Autodesk Inventor part; units mm, degrees
ref_plane "YZ Plane" through (0, 0, 0) normal (1, 0, 0) x (0, 1, 0)
ref_plane "XZ Plane" through (0, 0, 0) normal (0, 1, 0) x (-1, 0, 0)
ref_plane "XY Plane" through (0, 0, 0) normal (0, 0, 1) x (1, 0, 0)
sketch "Sketch1" plane through (0, 0, 0) normal (0, 1, 0) x (-1, 0, 0)
  circle A0 centre (-34.3765, 114.6665) radius 1.6
  circle A1 centre (-34.8464, 1.7591) radius 1.6
  arc A2 (-53.1019, 117.2341) -> (-38.3819, -1.7764) centre (30.561, 67.1665) ccw
  line L0 (-34.3765, 119.6665) -> (-48.8115, 119.6665)
  arc A3 (-38.3819, -1.7764) -> (-36.4764, -3.6306) centre (30.561, 67.1665) ccw
  line L1 (-33.0386, -5) -> (-21.9122, -5)
  line L2 (-16.9122, 0.0037) -> (-16.9963, 114.6702)
  line L3 (-21.9963, 119.6665) -> (-34.3765, 119.6665)
  arc A4 (-48.8115, 119.6665) -> (-53.1019, 117.2341) centre (-48.8115, 114.6665) ccw
  arc A5 (-36.4764, -3.6306) -> (-33.0386, -5) centre (-33.0386, 0) ccw
  circle A6 centre (-22.239, 104.2134) radius 1.25
  circle A7 centre (-53.239, 104.2134) radius 1.25
  circle A8 centre (-53.239, 29.2134) radius 1.25
  circle A9 centre (-22.239, 29.2134) radius 1.25
  line L4 (-24.639, 102.8634) -> (-24.639, 30.5634)
  line L5 (-24.639, 30.5634) -> (-51.939, 30.5634)
  line L6 (-51.939, 30.5634) -> (-51.939, 102.8634)
  line L7 (-51.939, 102.8634) -> (-24.639, 102.8634)
  arc A10 (-21.9122, -5) -> (-16.9122, 0.0037) centre (-21.9122, 0) ccw
  arc A11 (-16.9963, 114.6702) -> (-21.9963, 119.6665) centre (-21.9963, 114.6665) ccw
  point P0 (0, 0)
extrude "Extrusion1" add sketch "Sketch1" along normal blind 3
properties part number "LCD Plate" material "Polycarbonate, Clear"
Geometry: final body of the model. Coordinates: model frame, mm. A direction names the side the tool comes from. Round coordinates to 2 decimals unless told otherwise and drop trailing zeros. Loops run counter-clockwise (first coordinate to the right, second up) from the corner with the lowest first, then second, coordinate; pieces in that order, holes last.
Q1. Section A-A on z = 98.5. Return loops of the section in (x, y).
Q2. Pull-direction query (Z, two-part tool) for faces 3 (the cylindrical face through (34.864, 1.479, -4.655)), 4 (the cylindrical face through (66.086, 1.479, 54.302)), 5 (the cylindrical face through (53.51, 1.479, 105.434)); classes: released by +Z, released by -Z, zero draft, split by the parting line, or undercut.
Q3. Material intervals for L1, parallel to X at y = 1.9, z = 30; L2, parallel to X at y = 1.55, z = 103.5; L3, parallel to Z at x = 32.5, y = 1.5, sorted ascending.
Q4. Section D-D on x = 61. Return loops of the section in (y, z), plus the area to 3 significant figures.
Q5. Pin query (flat end, axial travel): P1, Ø3, axis at x = 53.24, z = 29.21, coming from the -Y side; P2, Ø0.9, axis at y = 2, z = 49, coming from the -X side; P3, Ø2, axis at x = 22.24, z = 104.21, coming from the -Y side; P4, Ø1.5, axis at y = 1, z = 20, coming from the +X side. Return the tip coordinate at first contact, or that it passes through.
Q6. Section C-C on x = 44. Return loops of the section in (y, z), plus the area to 3 significant figures.
Q7. Access query for faces 1 (the flat face through (51.939, 1, 66)), 2 (the flat face through (53, 3, 58)). Directions: +Z, -Z, +X, -X, +Y, -Y. A direction counts if a zero-diameter tool reaches every point of the face in a straight line with its end or side. Return the directions, or none.
Q8. Section B-B on y = 0.8. Return loops of the section in (x, z), plus the area to 3 significant figures.
Evaluation:
1. outline: (16.98, 0) - (24.64, 0) - (24.64, 3) - (16.98, 3) - close; (51.94, 0) - (61.77, 0) - (61.77, 3) - (51.94, 3) - close
2. face 3: released by -Z
2. face 4: split by the parting line
2. face 5: undercut
3. L1: x = 16.93 to 21.27, 23.21 to 52.27, 54.21 to 59.58
3. L2: x = 16.99 to 21.21, 23.27 to 52.21, 54.27 to 59.92
3. L3: z = -5 to 30.56, 102.86 to 119.67
4. outline: (0, 33.66) - (3, 33.66) - (3, 100.68) - (0, 100.68) - close
4. area: 201 mm2
5. P1: stops at y = 0
5. P2: stops at x = 16.95
5. P3: passes through
5. P4: stops at x = 55.18
6. outline: (0, 4.34) - (3, 4.34) - (3, 30.56) - (0, 30.56) - close; (0, 102.86) - (3, 102.86) - (3, 119.67) - (0, 119.67) - close
6. area: 129 mm2
7. face 1: +Y, -Y
7. face 2: +Z, -Z, +X, -X, +Y
8. outline: (16.91, 0) arc R5 ccw to (21.91, -5) - (33.04, -5) arc R5 ccw to (36.48, -3.63) arc R97.37 ccw to (38.38, -1.78) arc R97.5 ccw to (53.1, 117.23) arc R5 ccw to (48.81, 119.67) - (22, 119.67) arc R5 ccw to (17, 114.67) - close; hole circle Ø2.5 at (22.24, 29.21); hole circle Ø2.5 at (22.24, 104.21); hole (24.64, 30.56) - (51.94, 30.56) - (51.94, 102.86) - (24.64, 102.86) - close; hole circle Ø3.2 at (34.38, 114.67); hole circle Ø3.2 at (34.85, 1.76); hole circle Ø2.5 at (53.24, 29.21); hole circle Ø2.5 at (53.24, 104.21)
8. area: 3,240 mm2
